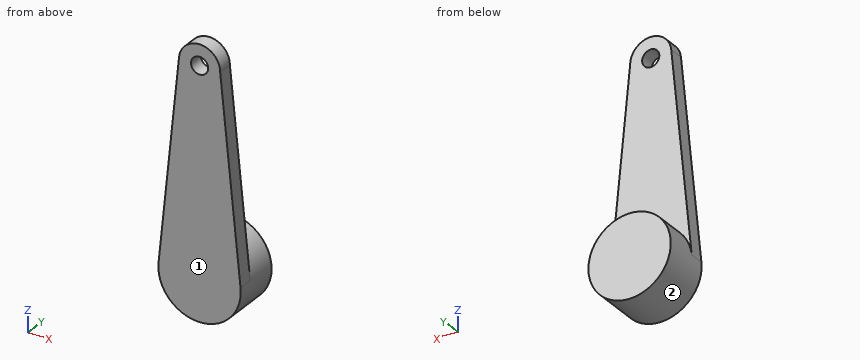
from build123d import *

# Parameters (mm, degrees)
SKETCH1_R           = 3
BOSS_EXTRUDE1_DEPTH = 3.5
SKETCH2_R           = 1.5
SKETCH2_R_2         = 0.625
BOSS_EXTRUDE2_DEPTH = 1.1


with BuildPart() as part:
    # Sketch1 → Boss-Extrude1 (new body)
    with BuildSketch(Plane(origin=(0, 0, 0), x_dir=(1, 0, 0), z_dir=(0, 1, 0))):
        Circle(SKETCH1_R)
    extrude(amount=BOSS_EXTRUDE1_DEPTH)

    # Sketch2 → Boss-Extrude2 (add)
    with BuildSketch(Plane(origin=(0, 0, 0), x_dir=(1, 0, 0), z_dir=(0, 1, 0))):
        with Locations((0, -15)):
            Circle(SKETCH2_R)
        with Locations((0, -15)):
            Circle(SKETCH2_R_2, mode=Mode.SUBTRACT)
        with BuildLine():
            ThreePointArc((2.984809248, -0.301519075), (-0.000763384, -2.999999903), (-2.984962311, -0.3))
            Line((-2.984962311, -0.3), (-1.492481156, -15.15))
            ThreePointArc((-1.492481156, -15.15), (-0.075094163, -13.50188089), (1.5, -15))
            Line((1.5, -15), (2.984809248, -0.301519075))
        make_face()
    extrude(amount=BOSS_EXTRUDE2_DEPTH)


solid = part.part
Model file for the job. Use its own axes, mm. Face numbers are marked on the shaded views. A direction names the side the tool comes from. Coordinates: 2 decimals unless noted, no trailing zeros. Order: outer loops, then holes, each group sorted by start corner. A loop starts at its lowest first (then second) coordinate and runs counter-clockwise, first axis right, second up. Notation, with made-up numbers: M -25,9.25 L 12,9.25 A7 cw 12,22.25 Z; hole C 36,-37 d10. An arc over 180 degrees is marked long. Return JSON: item names as keys, results as strings.
1. Drill centre lines: probe 1 along Z at (x, y) = (0, 0.65) (3 decimals); probe 2 along Y at (x, z) = (1.1, 13.5); probe 3 along X at (y, z) = (0.3, 15) (3 decimals). Where is each one in solid material? Low to high.
Ans:
{"probe 1": "-3 to 14.375, 15.625 to 16.5", "probe 2": "0 to 1.1", "probe 3": "-1.508 to -0.625, 0.625 to 1.5"}
2. Saw through at C-C (z = 9.5). Give the cut face in (x, y), and give its area (3 significant figures).
Ans:
{"outline": "M -2.06,0 L 2.06,0 L 2.06,1.1 L -2.06,1.1 Z", "area": "4.53 mm^2"}
3. Tool access for the marked faces 1 and 2: list every direction of +Z, -Z, +X, -X, +Y, -Y with a clear straight run to the whole face (end or side of a thin tool).
Ans:
{"face 1": "+Z, -Z, +X, -X, -Y", "face 2": "+Y"}
4. Flat gauge pins, fed straight in: pin 1 (1.5 mm diameter, centred on y = 2, z = 10.5, fed in from -X); pin 2 (1.8 mm diameter, centred on x = -0.5, z = 7.5, fed in from +Y). Where does each tip first touch, or does it go through?
Ans:
{"pin 1": "through", "pin 2": "y = 1.1"}
5. Saw through at B-B (y = 2.6). Give the cut face in (x, z).
Ans:
{"outline": "C 0,0 d6"}
6. Saw through at D-D (x = 2.45). Give the cut face in (y, z), and give its area (3 significant figures).
Ans:
{"outline": "M 0,-1.73 L 3.5,-1.73 L 3.5,1.73 L 1.1,1.73 L 1.1,5.6 L 0,5.6 Z", "area": "16.4 mm^2"}
7. Saw through at A-A (x = 0). Give the cut face in (y, z) (3 decimals).
Ans:
{"outline": "M 0,-3 L 3.5,-3 L 3.5,3 L 1.1,3 L 1.1,14.375 L 0,14.375 Z; M 0,15.625 L 1.1,15.625 L 1.1,16.5 L 0,16.5 Z"}
